Autodesk Fusion 360 part; units mm, degrees
sketch "Sketch1" plane through (0, 0, 0) normal (0, 1, 0) x (1, 0, 0) in component "Component"
  line L0 (0, 0) -> (40, 0)
  line L1 (40, 0) -> (40, -40)
  line L2 (40, -40) -> (0, -40)
  line L3 (0, -40) -> (0, 0)
  line L4 (0, -40) -> (40, 0)
  dimension "d1" = 40
sketch "Sketch2" plane through (0, 0, 0) normal (0, 0, 1) x (1, 0, 0) in component "Component"
  line L0 (0, 0) -> (40, 0)
  line L1 (40, 0) -> (40, 40)
  line L2 (40, 40) -> (0, 40)
  line L3 (0, 40) -> (0, 0)
  line L4 (0, 40) -> (40, 0)
  circle A0 centre (10, 10) radius 1.5
  dimension "d4" = 3
sketch "Sketch3" plane through (0, 0, 0) normal (1, 0, 0) x (0, 0, -1) in component "Component"
  line L0 (0, 0) -> (-40, 0)
  line L1 (-40, 0) -> (-40, 40)
  line L2 (-40, 40) -> (0, 40)
  line L3 (0, 40) -> (0, 0)
sketch "Sketch4" plane through (0, 0, 0) normal (1, 0, 0) x (0, 0, -1) in component "Component"
  line L0 (-40, 0) -> (0, 0)
  line L1 (0, 0) -> (0, 40)
  line L2 (0, 40) -> (-40, 40)
  line L3 (-40, 40) -> (-40, 0)
  line L4 (-40, 0) -> (0, 40)
  point P0 (-40, 0)
  point P1 (0, 40)
sketch "Sketch5" plane through (0, 0, 0) normal (1, 0, 0) x (0, 0, -1) in component "Component"
  line L0 (0, 40) -> (0, 0)
  circle A0 centre (-10, 10) radius 1.5
  point P0 (-40, 40)
  dimension "d3" = 3
sketch "Sketch6" plane through (0, 0, 0) normal (0, 1, 0) x (1, 0, 0) in component "Component"
  line L0 (0, 0) -> (40, -40)
  line L1 (0, 0) -> (0, -40)
  circle A0 centre (10, -10) radius 1.5
  point P0 (40, -40)
  dimension "d2" = 3
extrude "Extrude1" add sketch "Sketch3" against normal blind 5 makes body 1 in component "Component"
extrude "Extrude2" add sketch "Sketch2" against normal blind 5 separate body contours L0 L3 L4 makes body 2 in component "Component"
extrude "Extrude3" cut sketch "Sketch4" against normal blind 12 contours L2 L3 L4 bodies 1 in component "Component"
extrude "Extrude4" cut sketch "Sketch5" against normal blind 9 bodies 1 in component "Component"
extrude "Extrude5" add sketch "Sketch1" against normal blind 5 separate body contours L0 L3 L4 makes body 3 in component "Component"
extrude "Extrude6" cut sketch "Sketch6" against normal blind 31 bodies 3 in component "Component"
sketch "Sketch7" plane through (0, 0, 0) normal (0, 0, -1) x (-1, 0, 0) in component "Component"
  line L0 (0, 0) -> (-40, 0)
  line L1 (-40, 0) -> (-40, -5)
  line L2 (-40, -5) -> (0, -5)
  line L3 (0, -5) -> (0, 0)
  line L4 (0, -5) -> (5, 0)
  line L5 (5, 0) -> (0, 0)
  line L6 (0, -5) -> (0, 0)
  line L7 (5, 0) -> (0, 0)
extrude "Extrude7" add sketch "Sketch7" against normal blind 40 contours L3 L4 L5 L6 L7 bodies 1 2 3 in component "Component"
sketch "Sketch8" plane through (0, 0, 0) normal (0, -1, 0) x (1, 0, 0) in component "Component"
  line L0 (40, 0) -> (0, 0)
  line L1 (0, 0) -> (0, -5)
  line L2 (0, -5) -> (40, -5)
  line L3 (40, -5) -> (40, 0)
  line L4 (-5, 0) -> (0, -5)
  line L5 (0, 0) -> (-5, 0)
  line L6 (0, -5) -> (0, 0)
  point P0 (-5, 0)
  point P1 (-5, 0)
extrude "Extrude8" add sketch "Sketch8" against normal blind 40 separate body contours L1 L4 L5 L6 makes body 4 in component "Component"
sketch "Sketch9" plane through (0, 0, 0) normal (1, 0, 0) x (0, 0, -1) in component "Component"
  line L0 (0, 0) -> (0, -5)
  line L1 (0, 0) -> (0, -5)
  line L2 (5, 0) -> (0, 0)
  line L3 (0, -5) -> (5, 0)
  point P0 (0, -5)
  point P1 (5, 0)
extrude "Extrude9" add sketch "Sketch9" along normal blind 40 separate body makes body 5 in component "Component"
move_face "OffsetFaces1" offset 5 1 faces at (-1.6667, 0, -1.6667) on bodies 4 in component "Component"
sketch "Sketch10" plane through (0, 0, 0) normal (0, 0, 1) x (1, 0, 0) in component "Component"
  line L0 (-5, -5) -> (0, -5)
  line L1 (0, -5) -> (0, 40)
  line L2 (0, 40) -> (-5, 40)
  line L3 (-5, 40) -> (-5, -5)
  line L4 (-5, 0.0489) -> (0, -5)
  line L5 (-5, -5) -> (-5, 0.0489)
extrude "Extrude10" cut sketch "Sketch10" against normal blind 17 contours L0 L3 L4 L5 bodies 4 in component "Component"
sketch "Sketch11" plane through (0, 0, 0) normal (1, 0, 0) x (0, 0, -1) in component "Component"
  line L0 (0, -5) -> (5, -5)
  line L1 (5, -5) -> (5, 40)
  line L2 (5, 40) -> (0, 40)
  line L3 (0, 40) -> (0, -5)
  line L4 (0, -5) -> (5, 0)
  line L5 (5, -5) -> (0, -5)
  line L6 (5, 0) -> (5, -5)
  point P0 (5, 0)
extrude "Extrude11" cut sketch "Sketch11" against normal blind 18 contours L0 L1 L4 L5 L6 bodies 4 in component "Component"
sketch "Sketch12" plane through (0, 0, 0) normal (0, 1, 0) x (1, 0, 0) in component "Component"
  line L0 (47, 2) -> (47, -47)
  line L1 (47, -47) -> (-2, -47)
  line L2 (-2, -47) -> (-2, 2)
  line L3 (-2, 2) -> (47, 2)
extrude "Extrude12" cut sketch "Sketch12" along normal blind 65 bodies 1 4 makes body 6 at (17.0332, 0, 17.0068) in component "Component"
extrude "Extrude13" cut sketch "Sketch12" against normal blind 2 bodies 4 5 6 in component "Component"
sketch "Sketch13" plane through (0, 0, -5) normal (0, 0, -1) x (-1, 0, 0) in component "Component"
  circle A0 centre (-10, 10) radius 1.5
  line L0 (-40, 0) -> (0, 0)
  line L1 (0, 0) -> (0, 40)
  line L2 (0, 40) -> (-40, 0)
  circle A1 centre (-10, 10) radius 3.5
  dimension "d33" = 7
extrude "Extrude14" cut sketch "Sketch13" against normal blind 1 contours A1 bodies 1 in component "Component"
sketch "Sketch14" plane through (-5, 0, 0) normal (-1, 0, 0) x (0, 0, 1) in component "Component"
  circle A0 centre (10, 10) radius 1.5
  line L0 (40, 0) -> (0, 40)
  line L1 (0, 40) -> (0, 0)
  line L2 (0, 0) -> (40, 0)
  circle A1 centre (10, 10) radius 3.5
  dimension "d36" = 7
extrude "Extrude15" cut sketch "Sketch14" against normal blind 1 contours A1 bodies 6 in component "Component"
sketch "Sketch15" plane through (0, -5, 0) normal (0, -1, 0) x (1, 0, 0) in component "Component"
  circle A0 centre (10, 10) radius 1.5
  line L0 (0, 40) -> (0, 0)
  line L1 (0, 0) -> (40, 0)
  line L2 (40, 0) -> (0, 40)
  circle A1 centre (10, 10) radius 3.5
  dimension "d39" = 7
extrude "Extrude16" cut sketch "Sketch15" against normal blind 1 contours A1 bodies 6 in component "Component"
sketch "Sketch16" plane through (40, 0, 0) normal (1, 0, 0) x (0, 0, -1) in component "Component"
  line L0 (2, 0) -> (2, -2)
  line L1 (2, -2) -> (0, -2)
  line L2 (0, -2) -> (0, -5)
  line L3 (0, -5) -> (5, 0)
  line L4 (5, 0) -> (2, 0)
  line L5 (0, -5) -> (5, -5)
  line L6 (5, -5) -> (5, 0)
extrude "Extrude17" add sketch "Sketch16" against normal blind 40 contours L3 L5 L6 bodies 5 1 4 6 in component "Component"
sketch "Sketch17" plane through (0, 0, 40) normal (0, 0, 1) x (1, 0, 0) in component "Component"
  line L0 (0, -2) -> (-2, -2)
  line L1 (-2, -2) -> (-2, 0)
  line L2 (-2, 0) -> (-5, 0)
  line L3 (-5, 0) -> (0, -5)
  line L4 (0, -5) -> (0, -2)
  line L5 (-5, 0) -> (0, -5)
  line L6 (-5, -5) -> (-5, 0)
  line L7 (0, -5) -> (-5, -5)
extrude "Extrude18" add sketch "Sketch17" against normal blind 40 contours L3 L5 L6 L7 bodies 5 in component "Component"
sketch "Sketch18" plane through (0, 40, 0) normal (0, 1, 0) x (-1, 0, 0) in component "Component"
  line L0 (2, -2) -> (0, -2)
  line L1 (0, -2) -> (0, -5)
  line L2 (0, -5) -> (5, 0)
  line L3 (5, 0) -> (2, 0)
  line L4 (2, 0) -> (2, -2)
  line L5 (5, 0) -> (5, -5)
  line L6 (5, -5) -> (0, -5)
  line L7 (5, 0) -> (0, -5)
extrude "Extrude19" add sketch "Sketch18" against normal blind 45 separate body contours L2 L5 L6 L7 makes body 7 in component "Component"
sketch "Sketch19" plane through (0, -5, 0) normal (0, -1, 0) x (1, 0, 0) in component "Component"
  line L0 (-5, 0) -> (-5, -5)
  line L1 (-5, -5) -> (0, -5)
  line L2 (0, -5) -> (-5, 0)
  line L3 (-5, 0) -> (0, 0)
  line L4 (0, 0) -> (0, -5)
  line L5 (0, -5) -> (-5, -5)
  line L6 (-5, -5) -> (-5, 0)
extrude "Extrude20" add sketch "Sketch19" against normal blind 3 contours L2 L3 L4 bodies 5 7 in component "Component"
component "Component" placed x (1, 0, 0) y (0, 1, 0) z (0, 0, 1) at (15.4578, -1.4684, -4.3289)
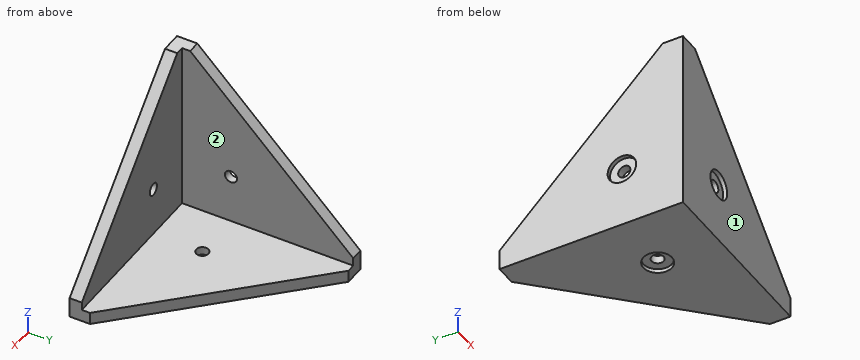
Source: CAD feature listing. Evaluate the final solid. Frame: model axes, mm. Face numbers are marked on the shaded views. A direction names the side the tool comes from. Round coordinates to 2 decimals unless told otherwise and drop trailing zeros. Write each loop counter-clockwise with the first axis right and the second up, starting at its lowest first coordinate (ties: lowest second). Pieces come first, ordered by that corner, then holes. Notation, with made-up numbers: M -0.5,-23.5 L 7.5,-23.5 A26 ccw 7.5,11.5 Z; hole C -22,-2.75 d5. An arc over 180 degrees is marked long. Use CSV: the item, a comma, the result in double quotes. Start each with the question number.
Q1. Cut plane A-A on x = 52.5. Output: boundary loops of the cut face in (y, z), plus the area to 3 significant figures.
Q2. Line query: line 1 (Z direction, x = 37.5, y = 5); line 2 (Y direction, x = 34.5, z = 4); line 3 (X direction, y = 29, z = -1). Output: solid intervals per line, ascending. Write a range as from..to.
Q3. Access query for the marked faces 1 and 2. Directions: +Z, -Z, +X, -X, +Y, -Y. A direction counts if a zero-diameter tool reaches every point of the face in a straight line with its end or side. Return the directions, or none.
Q4. First-contact query: P1, Ø3, axis at y = 25, z = 1, coming from the +X side; P2, Ø10, axis at x = 41.5, y = 19, coming from the +Z side; P3, Ø3.5, axis at x = 25.5, y = 8.5, coming from the -Z side. Flat tips, straight axial feed; report the tip coordinate or a pass-through.
Q5. Cut plane B-B on y = 30. Output: boundary loops of the cut face in (x, z).
Results found:
1,outline,"M -6.47,-9.33 L 1.49,-9.33 L 1.49,-6.33 L -3.47,-6.33 L -3.47,-1.37 L -6.47,-1.37 Z"
1,area,"38.7 mm^2"
2,line 1,"-9.33..-6.33"
2,line 2,"-6.47..-3.47"
2,line 3,"10.46..13.46"
3,face 1,"+Z, -Z, +X, -X, -Y"
3,face 2,"+Z, +X, +Y"
4,P1,"x = 13.46"
4,P2,"z = -6.33"
4,P3,"z = -8.33"
5,outline,"M 10.46,-9.33 L 23.99,-9.33 L 23.99,-6.33 L 13.46,-6.33 L 13.46,4.2 L 10.46,4.2 Z"
